The listing builds one solid part. Answer for the finished solid, in the listing's coordinates (mm). Face numbers are marked on the shaded views. A direction names the side the tool comes from. Give positions to 0.01 mm unless a question says otherwise; leave off trailing zeros. Loops run counter-clockwise (first coordinate to the right, second up) from the corner with the lowest first, then second, coordinate; pieces in that order, holes last. Notation, with made-up numbers: (-39, 52) -> (-14, 52) arc R36 ccw to (-14, 87) -> close; hole circle Ø10 at (47, -17). An arc over 180 degrees is marked (long way). One line per question, with ' | ' between items. Start each with the question number.
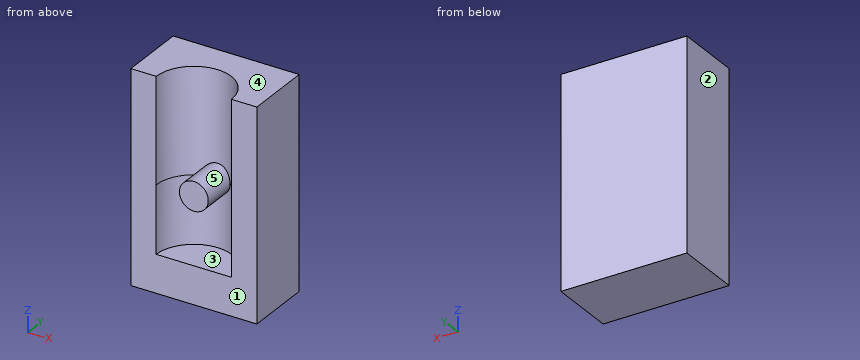
from build123d import *

# Parameters (mm, degrees)
F0_W          = 46.853558
F0_H          = 78.02628
F1_DEPTH      = 25
F2_R          = 13.971362
F3_DEPTH      = 42.8
F3_DEPTH_BACK = 25
F4_R          = 5.361649
F5_DEPTH      = 22.4


with BuildPart() as f1:
    # F0 (on Front) → F1 (new body)
    with BuildSketch(Plane.XZ):
        Rectangle(F0_W, F0_H)
    extrude(amount=-F1_DEPTH)

    # F2 (on Top) → F3 (cut, two sides)
    with BuildSketch(Plane.XY) as f3_sk:
        Circle(F2_R)
    extrude(amount=F3_DEPTH, mode=Mode.SUBTRACT)
    extrude(f3_sk.sketch, amount=-F3_DEPTH_BACK, mode=Mode.SUBTRACT)

    # F4 (on Front) → F5 (join)
    with BuildSketch(Plane.XZ):
        Circle(F4_R)
    extrude(amount=-F5_DEPTH)


solid = f1.part
1. The part is cut by section D-D (z = -4). Write down the section's boundary in (x, y), plus the area to 3 significant figures.
2. The part is cut by section C-C (z = 18). Write down the section's boundary in (x, y), plus the area to 3 significant figures.
3. For the marked faces 4 and 5, determine the directions among +Z, -Z, +X, -X, +Y, -Y from which every point of the face is accessible in a straight line to the end or side of a thin tool.
4. Each of these flat-tipped pins is pushed along its axis until it touches: pin 1 Ø7 at (x, y) = (-3, 5.5) entering from +Z; pin 2 Ø1.5 at (x, y) = (9.5, 9) entering from +Z. Where does it stop, or does it pass through?
5. The part is cut by section B-B (x = 0). Write down the section's boundary in (y, z), plus the area to 3 significant figures.
6. The part is cut by section A-A (y = 8.75). Write down the section's boundary in (x, z).
7. Determine the mould class of the marked faces 1, 2 and 3 for opening direction X: released by +X, released by -X, zero draft, split by the parting line, or undercut.
8. Straight lines are drawn through the part: L1, parallel to X at y = 3.75, z = -3; L2, parallel to X at y = 7, z = -0.5; L3, parallel to X at y = 11.5, z = -10.5. For each, find the intervals that lie inside material, in ascending order.
Check sheet entries:
1) outline: (-23.43, 0) -> (-13.97, 0) arc R13.97 cw to (-3.57, 13.51) -> (-3.57, 0) -> (3.57, 0) -> (3.57, 13.51) arc R13.97 cw to (13.97, 0) -> (23.43, 0) -> (23.43, 25) -> (-23.43, 25) -> close | area: 963 mm^2
2) outline: (-23.43, 0) -> (-13.97, 0) arc R13.97 cw to (13.97, 0) -> (23.43, 0) -> (23.43, 25) -> (-23.43, 25) -> close | area: 865 mm^2
3) face 4: +Z, +X, -X, +Y, -Y | face 5: -Y
4) pin 1: stops at z = 5.36 | pin 2: stops at z = -25
5) outline: (0, -39.01) -> (25, -39.01) -> (25, 39.01) -> (13.97, 39.01) -> (13.97, 5.36) -> (0, 5.36) -> (0, -5.36) -> (13.97, -5.36) -> (13.97, -25) -> (0, -25) -> close | area: 1,210 mm^2
6) outline: (-23.43, -39.01) -> (23.43, -39.01) -> (23.43, 39.01) -> (10.89, 39.01) -> (10.89, -25) -> (-10.89, -25) -> (-10.89, 39.01) -> (-23.43, 39.01) -> close; circle Ø10.72 at (0, 0)
7) face 1: zero draft | face 2: released by -X | face 3: undercut
8) L1: x = -23.43 to -13.46, -4.44 to 4.44, 13.46 to 23.43 | L2: x = -23.43 to -12.09, -5.34 to 5.34, 12.09 to 23.43 | L3: x = -23.43 to -7.93, 7.93 to 23.43
